Input: part model. Units: mm. Frame: model coordinates. Face numbers are marked on the shaded views. A direction names the side the tool comes from. Round coordinates to 2 decimals unless told otherwise and drop trailing zeros. Write each loop counter-clockwise with the first axis right and the second up, starting at its lowest first coordinate (ties: lowest second). Pieces come first, ordered by that corner, then holes. Notation, with made-up numbers: (64, 76) - (78, 76) arc R15 cw to (78, 93) - close; hole circle Ø9 at (43.25, 21). An arc over 180 degrees is marked (long way). Use one line per item in the form item = value.
```python
from build123d import *

# Parameters (mm, degrees)
F0_R     = 7.112
F0_R_2   = 38.1
F1_DEPTH = 12.7
F0_R_3   = 21.463
F2_DEPTH = 31.75
F4_START = -25.4
F4_DEPTH = 31.75


with BuildPart() as f1:
    # F0 (on Front) → F1 (new body)
    with BuildSketch(Plane.XZ):
        with BuildLine():
            ThreePointArc((12.7, 63.1597938122), (0, 69.596), (-12.7, 63.1597938122))
            Line((-12.7, 63.1597938122), (-49.6977319514, 12.7))
            ThreePointArc((-49.6977319514, 12.7), (-53.8547827604, 0), (-49.6977319514, -12.7))
            Line((-49.6977319514, -12.7), (-12.7, -63.1597938122))
            ThreePointArc((-12.7, -63.1597938122), (0, -69.596), (12.7, -63.1597938122))
            Line((12.7, -63.1597938122), (49.6977319514, -12.7))
            ThreePointArc((49.6977319514, -12.7), (53.8547827604, 0), (49.6977319514, 12.7))
            Line((49.6977319514, 12.7), (12.7, 63.1597938122))
        make_face()
        with Locations((0, -53.848)):
            Circle(F0_R, mode=Mode.SUBTRACT)
        Circle(F0_R_2, mode=Mode.SUBTRACT)
        with Locations((0, 53.848)):
            Circle(F0_R, mode=Mode.SUBTRACT)
    extrude(amount=F1_DEPTH)

    # F0 (on Front) → F2 (join)
    with BuildSketch(Plane.XZ):
        Circle(F0_R_2)
        Circle(F0_R_3, mode=Mode.SUBTRACT)
    extrude(amount=F2_DEPTH)

    # F3 (on Right) → F4 (cut)
    with BuildSketch(Plane.YZ.offset(F4_START)):
        with BuildLine():
            Line((-2.0067014742, -12.7), (-2.0067014742, 12.7))
            ThreePointArc((-2.0067014742, 12.7), (-5.8167014742, 16.51), (-9.6267014742, 12.7))
            Line((-9.6267014742, 12.7), (-9.6267014742, -12.7))
            ThreePointArc((-9.6267014742, -12.7), (-5.8167014742, -16.51), (-2.0067014742, -12.7))
        make_face()
    extrude(amount=-F4_DEPTH, mode=Mode.SUBTRACT)


solid = f1.part
```
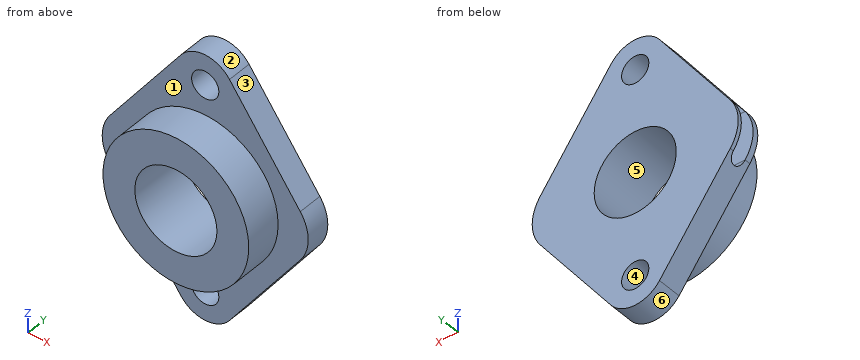
(1) Cut plane C-C on y = -5.5. Output: boundary loops of the cut face in (x, z), then the cut area to 3 significant figures.
Derived:
outline = (-46.91, -16.5) - (-12.7, -63.16) arc R15.75 ccw to (12.7, -63.16) - (49.7, -12.7) arc R21.48 ccw to (49.7, 12.7) - (12.7, 63.16) arc R15.75 ccw to (-12.7, 63.16) - (-46.91, 16.5) - (-25.4, 16.5) - (-25.4, -16.5) - close; hole circle Ø42.93 at (0, 0); hole circle Ø14.22 at (0, -53.85); hole circle Ø14.22 at (0, 53.85)
area = 6,570 mm^2
(2) Material intervals for L1, parallel to Z at x = 0, y = -6.5; L2, parallel to Z at x = 0, y = -14; L3, parallel to Y at x = -20.5, z = 39.5, sorted ascending.
Derived:
L1 = -69.6 to -60.96, -46.74 to -21.46, 21.46 to 46.74, 60.96 to 69.6
L2 = -38.1 to -21.46, 21.46 to 38.1
L3 = -12.7 to 0
(3) Access query for the marked faces 1 and 2. Directions: +Z, -Z, +X, -X, +Y, -Y. A direction counts if a zero-diameter tool reaches every point of the face in a straight line with its end or side. Return the directions, or none.
Derived:
face_1 = -Y
face_2 = +Z, +Y, -Y
(4) Cut plane D-D on z = -24.5. Output: boundary loops of the cut face in (x, y).
Derived:
outline = (-41.05, -12.7) - (-29.18, -12.7) - (-29.18, -31.75) - (29.18, -31.75) - (29.18, -12.7) - (41.05, -12.7) - (41.05, 0) - (-41.05, 0) - close
(5) Cut plane B-B on z = 0. Output: boundary loops of the cut face in (x, y), then the cut area to 3 significant figures.
Derived:
outline = (-53.85, -12.7) - (-38.1, -12.7) - (-38.1, -31.75) - (-21.46, -31.75) - (-21.46, 0) - (-53.85, 0) - (-53.85, -2.01) - (-25.4, -2.01) - (-25.4, -9.63) - (-53.85, -9.63) - close; (21.46, -31.75) - (38.1, -31.75) - (38.1, -12.7) - (53.85, -12.7) - (53.85, 0) - (21.46, 0) - close
area = 1,240 mm^2
(6) First-contact query: pin 1 Ø3 at (x, z) = (-23, 43) entering from -Y; pin 2 Ø4 at (y, z) = (-23, -32) entering from -X; pin 3 Ø4 at (x, y) = (-1, -25.5) entering from -Z. Flat tips, straight axial feed; report the tip coordinate or a pass-through.
Derived:
pin_1 = -12.7
pin_2 = -23.49
pin_3 = -38.1
(7) Draft query along X for the marked faces 3, 4, 5 and 6. Return one class per face: released by +X, released by -X, zero draft, split by the parting line, or undercut.
Derived:
face_3 = released by +X
face_4 = undercut
face_5 = undercut
face_6 = split by the parting line
(8) Cut plane A-A on x = 0. Output: boundary loops of the cut face in (y, z), then the cut area to 3 significant figures.
Derived:
outline = (-31.75, -38.1) - (-12.7, -38.1) - (-12.7, -46.74) - (0, -46.74) - (0, -21.46) - (-31.75, -21.46) - close; (-31.75, 21.46) - (0, 21.46) - (0, 46.74) - (-12.7, 46.74) - (-12.7, 38.1) - (-31.75, 38.1) - close; (-12.7, -69.6) - (0, -69.6) - (0, -60.96) - (-12.7, -60.96) - close; (-12.7, 60.96) - (0, 60.96) - (0, 69.6) - (-12.7, 69.6) - close
area = 1,500 mm^2
